from build123d import *

# Parameters (mm, degrees)
F0_R     = 6.35
F0_R_2   = 3.175
F2_DEPTH = 6.35
F1_R     = 3.175
F3_DEPTH = 97.100738786


with BuildPart() as f2:
    # F0 (on Right) → F2 (new body, symmetric)
    with BuildSketch(Plane.YZ):
        Circle(F0_R)
        Circle(F0_R_2, mode=Mode.SUBTRACT)
    extrude(amount=F2_DEPTH, both=True)



with BuildPart() as f2b:
    # F0 (on Right) → F2, piece 2 (new body, symmetric)
    with BuildSketch(Plane.YZ):
        with Locations((101.6, 0)):
            Circle(F0_R)
        with Locations((101.6, 0)):
            Circle(F0_R_2, mode=Mode.SUBTRACT)
    extrude(amount=F2_DEPTH, both=True)


with BuildPart() as f2_1:
    add(f2.part)

    add(f2b.part)  # F3 merges F2b
    # F1 (on Front) → F3 (join, up to face)
    with BuildSketch(Plane.XZ):
        Circle(F1_R)
    extrude(amount=-F3_DEPTH)


solid = f2_1.part
Geometry: final body of the model. Coordinates: model frame, mm. A direction names the side the tool comes from. Give positions to 0.01 mm unless a question says otherwise; leave off trailing zeros. Loops run counter-clockwise (first coordinate to the right, second up) from the corner with the lowest first, then second, coordinate; pieces in that order, holes last. Notation, with made-up numbers: M 62,44 L 77,44 A28 cw 77,72 Z; hole C -35.5,-8 d10. An arc over 180 degrees is marked long. Put each result on its own line as item: value. Start each with the question number.
1) Access query for faces 1 (the flat face through (0, 0, 0)), 2 (the cylindrical face through (-0.69, 50.17, -3.1)), 3 (the flat face through (-6.35, 100, 3)). Directions: +Z, -Z, +X, -X, +Y, -Y. A direction counts if a zero-diameter tool reaches every point of the face in a straight line with its end or side. Return the directions, or none.
2) Cut plane C-C (x = 4.75). Output: boundary loops of the cut face in (y, z) (3 decimals), then the cut area to 3 significant figures.
3) Pull-direction query (Y, two-part tool) for faces 4 (the flat face through (6.35, 100, 3)), 5 (the cylindrical face through (0.089, -6.344, 0.279)), 6 (the cylindrical face through (-3.174, 1.212, 0.07)); classes: pulls with the +Y half, pulls with the -Y half, needs draft (parallel to the pull), parting line crosses it, or undercut.
4) Contact query for flat-ended pins moving along their axis: pin 1 (6 mm diameter, centred on x = 3.5, y = 15, fed in from +Z); pin 2 (2 mm diameter, centred on x = 0.5, y = 68, fed in from -Z) (3 decimals); pin 3 (5.5 mm diameter, centred on y = 0, z = 0, fed in from +X) (3 decimals). Output: stop coordinate, or through.
5) Cut plane A-A (z = 0). Output: boundary loops of the cut face in (x, y) (3 decimals).
6) Cut plane B-B (y = 101.6). Output: boundary loops of the cut face in (x, z) (3 decimals).
7) Cut plane D-D (x = -2). Output: boundary loops of the cut face in (y, z) (3 decimals).
8) Ray query, line 1 along Y through (x, z) = (2, -2); line 2 along Y through (x, z) = (-5.25, 3.75); line 3 along Y through (x, z) = (-3.75, 1.5). Return the intervals inside material, ascending.
Verdict:
1. face 1: +X, -X
1. face 2: none
1. face 3: +Z, -Z, -X, +Y, -Y
2. outline: C 0,0 d12.7; C 101.6,0 d12.7; hole C 0,0 d6.35; hole C 101.6,0 d6.35
2. area: 190 mm2
3. face 4: needs draft
3. face 5: undercut
3. face 6: undercut
4. pin 1: z = 3.14
4. pin 2: z = -3.175
4. pin 3: x = 3.175
5. outline: M -6.35,-6.35 L 6.35,-6.35 L 6.35,-3.175 L -6.35,-3.175 Z; M -6.35,3.175 L -3.175,3.175 L -3.175,0 L 3.175,0 L 3.175,3.175 L 6.35,3.175 L 6.35,6.35 L 3.175,6.35 L 3.175,95.25 L 6.35,95.25 L 6.35,98.425 L -6.35,98.425 L -6.35,95.25 L -3.175,95.25 L -3.175,6.35 L -6.35,6.35 Z; M -6.35,104.775 L 6.35,104.775 L 6.35,107.95 L -6.35,107.95 Z
6. outline: M -6.35,-6.35 L 6.35,-6.35 L 6.35,-3.175 L -6.35,-3.175 Z; M -6.35,3.175 L 6.35,3.175 L 6.35,6.35 L -6.35,6.35 Z
7. outline: M 5.852,-2.466 L 95.748,-2.466 A6.35 ccw long 95.748,2.466 L 5.852,2.466 A6.35 ccw long Z; hole M 0,-2.466 L 0,2.466 L 2,2.466 A3.175 ccw long 2,-2.466 Z; hole C 101.6,0 d6.35
8. line 1: -6.03 to -2.47, 0 to 99.13, 104.07 to 107.63
8. line 2: -5.12 to 5.12, 96.48 to 106.72
8. line 3: -6.17 to -2.8, 2.8 to 6.17, 95.43 to 98.8, 104.4 to 107.77
